Could you check a few things on this drawing? It's one solid part, dimensions in mm from its lowest x, y, z. A direction names the side the tool comes from. Coordinates: 2 decimals unless noted, no trailing zeros. Write each loop counter-clockwise with the first axis right and the second up, starting at its lowest first coordinate (ties: lowest second). Pieces come first, ordered by that corner, then holes. Notation, with made-up numbers: (-11.5, -17) - (-1.5, -17) arc R7 ccw to (-1.5, -12) - close; hole circle Ø3 at (-25.5, 83.5). An arc over 180 degrees is marked (long way). Write each question's results on one line, items separated by ' | '. Start each with the question number.
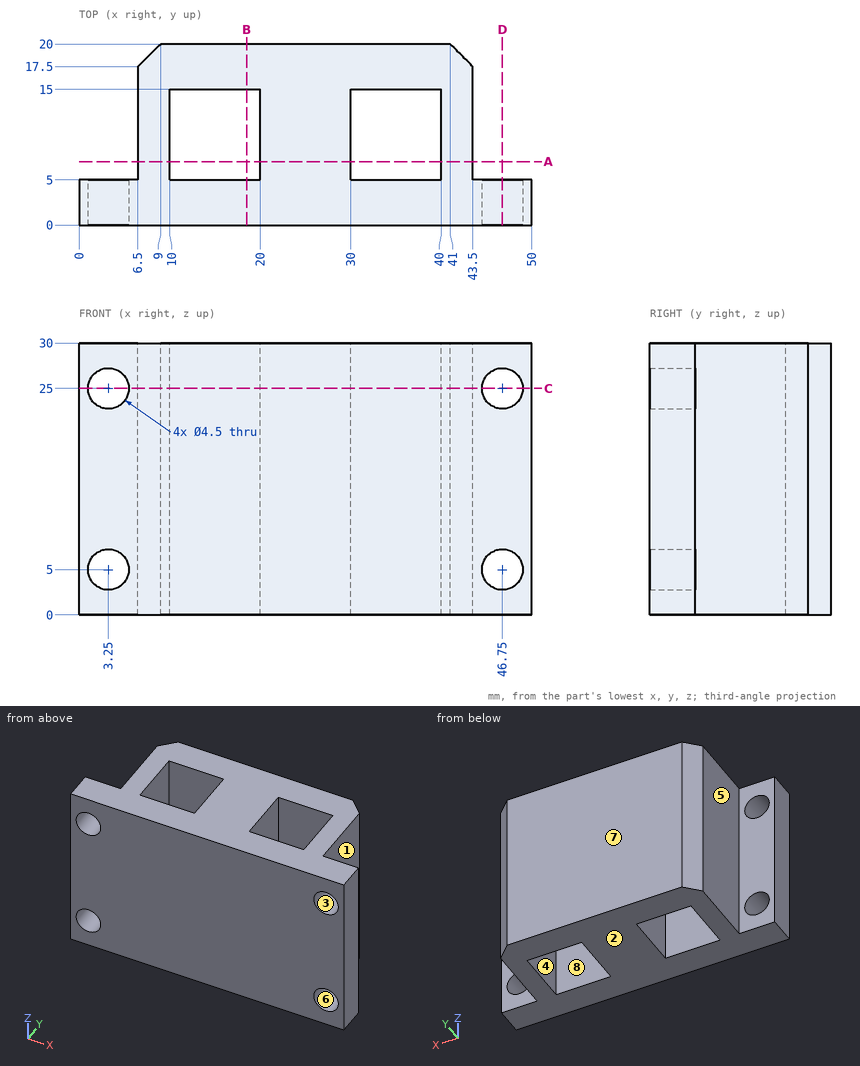
Q1. If we section it at A-A (y = 7): Please give me the cut outline in (x, z).
Q2. For the marked faces 1, 2, 3, 4 and 5, which set-ups out of +Z, -Z, +X, -X, +Y, -Y let a thin tool reach every point of the face, with its end or its side?
Q3. If we section it at D-D (x = 46.75): Please give me the cut outline in (y, z).
Q4. If we section it at C-C (z = 25): Please give me the cut outline in (x, y), then the cut area to 3 significant figures.
Q5. I'm going to push flat-ended pins straight in: pin 1 Ø2 at (y, z) = (10.5, 4.5) entering from +X; pin 2 Ø1.5 at (x, z) = (42.5, 17) entering from +Y; pin 3 Ø3 at (x, z) = (3.5, 14) entering from +Y; pin 4 Ø4 at (x, z) = (46.75, 25) entering from -Y. Where does each tip first touch, or does it pass through?
Q6. I need wall thicknesses on line 1 along X through (y, z) = (2.9, 25); line 2 along X through (y, z) = (5.25, 25.5); line 3 along Z through (x, y) = (3.25, 3). Which ranges of each line are inside material? Lowest first, please. Write a range as from..to.
Q7. Thinking about a two-plate mould opening in Y: for the marked faces 6, 7 and 8, which applies, pulls with the +Y half, pulls with the -Y half, needs draft (parallel to the pull), parting line crosses it, or undercut?
Q8. If we section it at B-B (x = 18.5): Please give me the cut outline in (y, z), then the cut area to 3 significant figures.
Answer list:
1) outline: (6.5, 0) - (10, 0) - (10, 30) - (6.5, 30) - close; (20, 0) - (30, 0) - (30, 30) - (20, 30) - close; (40, 0) - (43.5, 0) - (43.5, 30) - (40, 30) - close
2) face 1: +Z, -Z, +X, +Y | face 2: -Z, +X, -X, +Y, -Y | face 3: +Y, -Y | face 4: +Z, -Z | face 5: +Z, -Z, -X, +Y
3) outline: (0, 0) - (5, 0) - (5, 2.75) - (0, 2.75) - close; (0, 7.25) - (5, 7.25) - (5, 22.75) - (0, 22.75) - close; (0, 27.25) - (5, 27.25) - (5, 30) - (0, 30) - close
4) outline: (0, 0) - (1, 0) - (1, 5) - (0, 5) - close; (5.5, 0) - (44.5, 0) - (44.5, 5) - (43.5, 5) - (43.5, 17.5) - (41, 20) - (9, 20) - (6.5, 17.5) - (6.5, 5) - (5.5, 5) - close; (49, 0) - (50, 0) - (50, 5) - (49, 5) - close; hole (10, 5) - (20, 5) - (20, 15) - (10, 15) - close; hole (30, 5) - (40, 5) - (40, 15) - (30, 15) - close | area: 554 mm2
5) pin 1: stops at x = 43.5 | pin 2: stops at y = 19.25 | pin 3: stops at y = 5 | pin 4: passes through
6) line 1: x = 0..1, 5.5..44.5, 49..50 | line 2: x = 6.5..10, 20..30, 40..43.5 | line 3: z = 0..2.75, 7.25..22.75, 27.25..30
7) face 6: needs draft | face 7: pulls with the +Y half | face 8: undercut
8) outline: (0, 0) - (5, 0) - (5, 30) - (0, 30) - close; (15, 0) - (20, 0) - (20, 30) - (15, 30) - close | area: 300 mm2
